from build123d import *

# Parameters (mm, degrees)
F0_R     = 2
F0_W     = 5
F0_H     = 51
F0_W_2   = 49.9
F0_H_2   = 70
F1_DEPTH = 2
F2_DEPTH = 6
F3_DEPTH = 13


with BuildPart() as f1:
    # F0 (on Top) → F1 (new body)
    with BuildSketch(Plane.XY):
        Polygon((-25.6, 35.5), (-32.8, 35.5), (-32.8, -35.5), (32.8, -35.5), (32.8, 35.5), (24.3, 35.5), (24.3, -34.5), (-25.6, -34.5), align=None)
        with Locations((-28.3, -31)):
            Circle(F0_R, mode=Mode.SUBTRACT)
        with Locations((30, -31)):
            Circle(F0_R, mode=Mode.SUBTRACT)
        with Locations((-28.3, 0)):
            Rectangle(F0_W, F0_H, mode=Mode.SUBTRACT)
        with Locations((-28.3, 31)):
            Circle(F0_R, mode=Mode.SUBTRACT)
        with Locations((30, 31)):
            Circle(F0_R, mode=Mode.SUBTRACT)
        with Locations((-0.65, 0.5)):
            Rectangle(F0_W_2, F0_H_2)
        with Locations((-28.3, 0)):
            Rectangle(F0_W, F0_H)
    extrude(amount=F1_DEPTH)

    # F0 (on Top) → F2 (join)
    with BuildSketch(Plane.XY):
        with Locations((-0.65, 0.5)):
            Rectangle(F0_W_2, F0_H_2)
    extrude(amount=F2_DEPTH)

    # F0 (on Top) → F3 (join)
    with BuildSketch(Plane.XY):
        with Locations((-28.3, 0)):
            Rectangle(F0_W, F0_H)
    extrude(amount=-F3_DEPTH)


solid = f1.part
Can you work these out from the model? Positions are in its coordinate system, mm. A direction names the side the tool comes from. Give positions to 0.01 mm unless a question says otherwise; leave off trailing zeros. Loops run counter-clockwise (first coordinate to the right, second up) from the corner with the lowest first, then second, coordinate; pieces in that order, holes last. Notation, with made-up numbers: (21, 8.5) -> (77, 8.5) arc R15 ccw to (77, 33.5) -> close; hole circle Ø8 at (67, 26.25). An arc over 180 degrees is marked (long way). Write item = value, one per line.
1) Will these pins go through, and if not, where does the flat tip stop? pin 1 (1.5 mm diameter, centred on x = -29, z = -6, fed in from +Y); pin 2 (2.5 mm diameter, centred on x = 30, y = 31, fed in from -Z); pin 3 (3 mm diameter, centred on y = -4.5, z = 4.5, fed in from +X); pin 4 (5 mm diameter, centred on y = -27, z = -10, fed in from +X).
Check result:
pin_1 = 25.5
pin_2 = through
pin_3 = 24.3
pin_4 = -25.8
2) Suppose I cut it at D-D on x = -15.5. Write out the boundary of the cut face in (y, z), then the cut area to 3 significant figures.
Check result:
outline = (-35.5, 0) -> (35.5, 0) -> (35.5, 6) -> (-34.5, 6) -> (-34.5, 2) -> (-35.5, 2) -> close
area = 422 mm2
3) For faces 1 (the flat face through (24.3, 0, 4)), 2 (the flat face through (-28, -25.5, -6)), 3 (the flat face through (-1, -34.5, 4)), 4 (the flat face through (-30.8, 0, -6)), 5 (the flat face through (-25.8, 0, -6)), which set-ups out of +Z, -Z, +X, -X, +Y, -Y let a thin tool reach every point of the face, with its end or its side?
Check result:
face_1 = +Z, +X, +Y, -Y
face_2 = -Z, +X, -X, -Y
face_3 = +Z, +X, -X, -Y
face_4 = -Z, -X, +Y, -Y
face_5 = -Z, +X, +Y, -Y
4) I need wall thicknesses on L1, parallel to Y at x = -28.3, z = 1.6; L2, parallel to X at y = -24.5, z = -5.25; L3, parallel to Z at x = 18, y = 19.5. Which ranges of each line are inside material? Lowest first, please. Write a range as from..to.
Check result:
L1 = -35.5..-33, -29..29, 33..35.5
L2 = -30.8..-25.8
L3 = 0..6
5) Suppose I cut it at C-C on y = 2.5. Write out the boundary of the cut face in (x, z), then the cut area to 3 significant figures.
Check result:
outline = (-32.8, 0) -> (-30.8, 0) -> (-30.8, -13) -> (-25.8, -13) -> (-25.8, 0) -> (32.8, 0) -> (32.8, 2) -> (24.3, 2) -> (24.3, 6) -> (-25.6, 6) -> (-25.6, 2) -> (-32.8, 2) -> close
area = 396 mm2
6) Suppose I cut it at A-A on y = -31. Write out the boundary of the cut face in (x, z).
Check result:
outline = (-32.8, 0) -> (-30.3, 0) -> (-30.3, 2) -> (-32.8, 2) -> close; (-26.3, 0) -> (28, 0) -> (28, 2) -> (24.3, 2) -> (24.3, 6) -> (-25.6, 6) -> (-25.6, 2) -> (-26.3, 2) -> close; (32, 0) -> (32.8, 0) -> (32.8, 2) -> (32, 2) -> close
7) Suppose I cut it at B-B on x = -28.3. Write out the boundary of the cut face in (y, z).
Check result:
outline = (-35.5, 0) -> (-33, 0) -> (-33, 2) -> (-35.5, 2) -> close; (-29, 0) -> (-25.5, 0) -> (-25.5, -13) -> (25.5, -13) -> (25.5, 0) -> (29, 0) -> (29, 2) -> (-29, 2) -> close; (33, 0) -> (35.5, 0) -> (35.5, 2) -> (33, 2) -> close
8) Thinking about a two-plate mould opening in X: for faces 6 (the flat face through (-1, 1, 6)), 7 (the cylindrical face through (-27.377, -32.774, 0.986)), 8 (the flat face through (32.8, 0, 1)), which applies, released by +X, released by -X, zero draft, split by the parting line, or undercut?
Check result:
face_6 = zero draft
face_7 = undercut
face_8 = released by +X
